Could you check a few things on this model? Use its own coordinates, in mm. Face numbers are marked on the shaded views. A direction names the side the tool comes from. Round coordinates to 2 decimals unless told otherwise and drop trailing zeros. Order: outer loops, then holes, each group sorted by start corner. A loop starts at its lowest first (then second) coordinate and runs counter-clockwise, first axis right, second up. Notation, with made-up numbers: (64.25, 19.25) -> (117.25, 19.25) arc R32 ccw to (117.25, 47.25) -> close; hole circle Ø10 at (84, 89.25). An arc over 180 degrees is marked (long way). One line per question, with ' | ' between items.
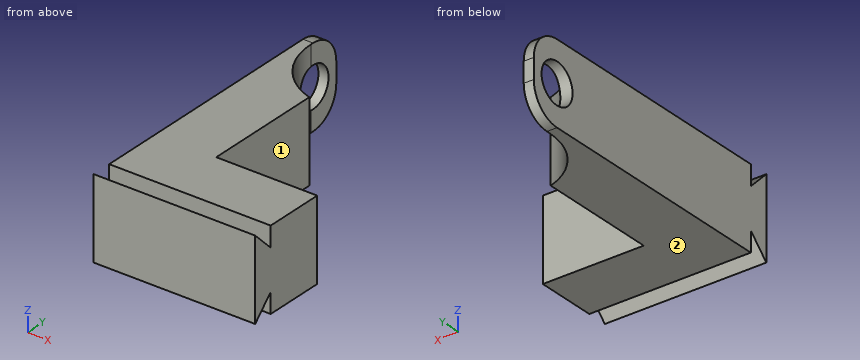
```python
from build123d import *

# Parameters (mm, degrees)
SKETCH1_W           = 8
SKETCH1_H           = 30
BOSS_EXTRUDE1_DEPTH = 6
SKETCH2_W           = 8
SKETCH2_H           = 10
CUT_EXTRUDE1_DEPTH  = 5
CUT_EXTRUDE2_REACH  = 18.643
SKETCH3_R           = 2
FILLET1_R           = 3
FILLET2_R           = 7
SKETCH4_W           = 8
SKETCH4_H           = 8
BOSS_EXTRUDE2_DEPTH = 10
CUT_EXTRUDE4_REACH  = 24.293


with BuildPart() as part:
    # Sketch1 → Boss-Extrude1 (new body)
    with BuildSketch(Plane(origin=(0, 0, 0), x_dir=(0, 0, -1), z_dir=(1, 0, 0))):
        Rectangle(SKETCH1_W, SKETCH1_H)
    extrude(amount=BOSS_EXTRUDE1_DEPTH)

    # Sketch2 → Cut-Extrude1 (cut)
    with BuildSketch(Plane(origin=(6, 0, 0), x_dir=(0, 0, -1), z_dir=(1, 0, 0))):
        with Locations((0, 10)):
            Rectangle(SKETCH2_W, SKETCH2_H)
    extrude(amount=-CUT_EXTRUDE1_DEPTH, mode=Mode.SUBTRACT)

    # Sketch3 → Cut-Extrude2 (cut, up to next)
    with BuildSketch(Plane.ZY, mode=Mode.PRIVATE) as cut_extrude2_sk1:
        with Locations((0, 12)):
            Circle(SKETCH3_R)
    cut_extrude2_tool1 = extrude(cut_extrude2_sk1.sketch, amount=-CUT_EXTRUDE2_REACH, mode=Mode.PRIVATE) & part.part
    add(cut_extrude2_tool1.solids().sort_by_distance((0, 12, 0))[0], mode=Mode.SUBTRACT)

    # Fillet1
    fillet1_edges = [part.edges().sort_by_distance(p)[0] for p in [
        (0.5, 15, 4),
        (0.5, 15, -4),
    ]]
    fillet(fillet1_edges, radius=FILLET1_R)

    # Fillet2
    # the kernel refuses this fillet: 7 mm, written as the material it adds along each edge
    with BuildSketch(Plane(origin=(1, 5, 4), x_dir=(0, 1, 0), z_dir=(0, 0, -1))) as fillet2_piece_1_section:
        with BuildLine():
            CenterArc((6.708203932, 7), FILLET2_R, 196.601549599, 73.398450401)
            Line((0, 5), (0, 0))
            Line((0, 0), (6.708203932, 0))
        make_face()
    fillet2_piece_1 = extrude(amount=8, mode=Mode.PRIVATE)
    fillet2_piece_1 = fillet2_piece_1 - Plane(origin=(1, 12, 0), x_dir=(0, 0, 1), z_dir=(-1, 0, 0)) * Cylinder(2, 43, mode=Mode.PRIVATE)
    add(fillet2_piece_1)

    # Sketch4 → Boss-Extrude2 (add)
    with BuildSketch(Plane(origin=(6, 0, 0), x_dir=(0, 0, -1), z_dir=(1, 0, 0))):
        with Locations((0, -11)):
            Rectangle(SKETCH4_W, SKETCH4_H)
    extrude(amount=BOSS_EXTRUDE2_DEPTH)

    # Sketch6 → Cut-Extrude4 (cut, up to next)
    with BuildSketch(Plane.ZY, mode=Mode.PRIVATE) as cut_extrude4_sk1:
        Polygon((4, -15), (4, -13), (2, -13), align=None)
    cut_extrude4_tool1 = extrude(cut_extrude4_sk1.sketch, amount=-CUT_EXTRUDE4_REACH, mode=Mode.PRIVATE) & part.part
    # Sketch6 → Cut-Extrude4 (cut, up to next)
    with BuildSketch(Plane.ZY, mode=Mode.PRIVATE) as cut_extrude4_sk2:
        Polygon((-4, -15), (-4, -13), (-2, -13), align=None)
    cut_extrude4_tool2 = extrude(cut_extrude4_sk2.sketch, amount=-CUT_EXTRUDE4_REACH, mode=Mode.PRIVATE) & part.part
    add(cut_extrude4_tool1.solids().sort_by_distance((0, -13.666667, 3.333333))[0], mode=Mode.SUBTRACT)
    add(cut_extrude4_tool2.solids().sort_by_distance((0, -13.666667, -3.333333))[0], mode=Mode.SUBTRACT)


solid = part.part
```
1. I want a section at D-D on y = -5. List the corners of the cut face in (x, z) for me, and give its area (3 significant figures).
From the geometry:
outline: (0, -4) -> (6, -4) -> (6, 4) -> (0, 4) -> close | area: 48.0 mm²
2. On a 3-axis mill with a long thin cutter (end or side, diameter ignored), from which of +Z, -Z, +X, -X, +Y, -Y can I reach the whole of each face in a straight line? I mean the marked faces 1 and 2. Say none if no direction works.
From the geometry:
face 1: +Z, -Z, +X, +Y | face 2: -Z, +X, -X, +Y, -Y
3. I want a section at B-B on x = 6.5. List the corners of the cut face in (y, z) for me, and give its area (3 significant figures).
From the geometry:
outline: (-15, -4) -> (-13, -2) -> (-13, -4) -> (-7, -4) -> (-7, 4) -> (-13, 4) -> (-13, 2) -> (-15, 4) -> close | area: 60.0 mm²
4. I want a section at A-A on z = 0. List the corners of the cut face in (x, y) for me, and give its area (3 significant figures).
From the geometry:
outline: (0, -15) -> (16, -15) -> (16, -7) -> (6, -7) -> (6, 5) arc R7 cw to (1.21, 10) -> (0, 10) -> close; (0, 14) -> (1, 14) -> (1, 15) -> (0, 15) -> close | area: 215 mm²
5. I'm going to push flat-ended pins straight in: pin 1 (2.5 mm diameter, centred on x = 12.5, z = 1.5, fed in from +Y); pin 2 (3.5 mm diameter, centred on y = 14, z = -0.5, fed in from +X); pin 3 (1.5 mm diameter, centred on x = 6, z = 2.5, fed in from +Y). Where does each tip first touch, or does it pass through?
From the geometry:
pin 1: stops at y = -7 | pin 2: stops at x = 1 | pin 3: stops at y = 5.27
6. I need wall thicknesses on probe 1 along Z at (x, y) = (0.7, 12); probe 2 along Y at (x, z) = (0.45, 0); probe 3 along Y at (x, z) = (10.75, -1). Which ranges of each line are inside material? Lowest first, please.
From the geometry:
probe 1: z = -4 to -2, 2 to 4 | probe 2: y = -15 to 10, 14 to 15 | probe 3: y = -15 to -7
7. I want a section at C-C on z = -3.25. List the corners of the cut face in (x, y) for me, and give its area (3 significant figures).
From the geometry:
outline: (0, -15) -> (16, -15) -> (16, -14.25) -> (0, -14.25) -> close; (0, -13) -> (16, -13) -> (16, -7) -> (6, -7) -> (6, 5) arc R7 cw to (1, 11.71) -> (1, 13.98) -> (0, 13.98) -> close | area: 198 mm²
